Read the model definition and answer for the solid it produces. Units are mm, in the model's axes. A direction names the side the tool comes from. Give positions to 0.01 mm unless a question says otherwise; leave off trailing zeros. Write each loop counter-clockwise with the first axis right and the second up, starting at its lowest first coordinate (ties: lowest second). Pieces come first, ordered by that corner, then holes. Notation, with made-up numbers: M -31,35 L -8,35 A16 cw -8,61 Z; hole C -20,-15 d4. An arc over 180 degrees is marked long. Write each question's results on one line, items separated by ' | '. Start each with the question number.
```python
from build123d import *

# Parameters (mm, degrees)
SKETCH1_W                                 = 50.8
SKETCH1_H                                 = 63.5
BOSS_EXTRUDE1_DEPTH                       = 12.065
SKETCH6_W                                 = 50.8
SKETCH6_H                                 = 12.065
BOSS_EXTRUDE2_DEPTH                       = 6.35
F_13_64_0_20313_DIAMETER_HOLE1_AT_2_COUNT = 2
F_13_64_0_20313_DIAMETER_HOLE1_AT_2_PITCH = 31.75
SKETCH12_W                                = 25.4
SKETCH12_H                                = 50.8
CUT_EXTRUDE7_DEPTH                        = 48.353291596
FILLET1_R                                 = 6.35
SKETCH13_R                                = 19.05
CUT_EXTRUDE8_DEPTH                        = 48.353291596
FILLET2_R                                 = 6.35


with BuildPart() as part:
    # Sketch1 → Boss-Extrude1 (new body)
    with BuildSketch(Plane.XY):
        Rectangle(SKETCH1_W, SKETCH1_H)
    extrude(amount=BOSS_EXTRUDE1_DEPTH)

    # Sketch6 → Boss-Extrude2 (add)
    with BuildSketch(Plane.XZ.offset(31.75)):
        with Locations((0, 6.0325)):
            Rectangle(SKETCH6_W, SKETCH6_H)
    boss_extrude2 = extrude(amount=BOSS_EXTRUDE2_DEPTH)

    # Sketch8 → 13_64 _0.20313_ Diameter Hole1 (revolve, cut)
    with BuildSketch(Plane(origin=(-15.875, -38.1, 6.0325), x_dir=(0, 0, -1), z_dir=(1, 0, 0))):
        Polygon((0, 0), (0, 16.790070783), (2.579751, 15.24), (2.579751, 0), align=None)
    f_13_64_0_20313_diameter_hole1 = revolve(axis=Axis((-15.875, -44.45, 6.0325), (0, 1, 0)), mode=Mode.SUBTRACT)

    # 13_64 _0.20313_ Diameter Hole1 at 2: 13_64 _0.20313_ Diameter Hole1 ×2
    with Locations(*[(i * F_13_64_0_20313_DIAMETER_HOLE1_AT_2_PITCH, 0, 0) for i in range(1, F_13_64_0_20313_DIAMETER_HOLE1_AT_2_COUNT)]):
        add(f_13_64_0_20313_diameter_hole1, mode=Mode.SUBTRACT)

    # Mirror2: Boss-Extrude2, 13_64 _0.20313_ Diameter Hole1 across plane
    add(boss_extrude2.mirror(Plane.ZX))
    add(f_13_64_0_20313_diameter_hole1.mirror(Plane.ZX), mode=Mode.SUBTRACT)

    # Mirror2 copy 1 sketch → Mirror2 copy 1 (revolve, cut)
    with BuildSketch(Plane(origin=(15.875, 38.1, 6.0325), x_dir=(0, 0, -1), z_dir=(1, 0, 0))):
        Polygon((0, 0), (0, -16.790070783), (2.579751, -15.24), (2.579751, 0), align=None)
    revolve(axis=Axis((15.875, 44.45, 6.0325), (0, 1, 0)), mode=Mode.SUBTRACT)

    # Sketch12 → Cut-Extrude7 (cut, through all)
    with BuildSketch(Plane.XY.offset(12.065)):
        Rectangle(SKETCH12_W, SKETCH12_H)
    extrude(amount=-CUT_EXTRUDE7_DEPTH, mode=Mode.SUBTRACT)

    # Fillet1
    fillet1_edges = [part.edges().sort_by_distance(p)[0] for p in [
        (-12.7, -25.4, 6.0325),
        (-12.7, 25.4, 6.0325),
        (12.7, 25.4, 6.0325),
        (12.7, -25.4, 6.0325),
    ]]
    fillet(fillet1_edges, radius=FILLET1_R)

    # Sketch13 → Cut-Extrude8 (cut, through all)
    with BuildSketch(Plane(origin=(0, 0, 0), x_dir=(-1, 0, 0), z_dir=(0, 0, -1))):
        Circle(SKETCH13_R)
    extrude(amount=-CUT_EXTRUDE8_DEPTH, mode=Mode.SUBTRACT)

    # Fillet2
    fillet2_edges = [part.edges().sort_by_distance(p)[0] for p in [
        (12.7, 14.199031657, 6.0325),
        (12.7, -14.199031657, 6.0325),
        (-12.7, 14.199031657, 6.0325),
        (-12.7, -14.199031657, 6.0325),
    ]]
    fillet(fillet2_edges, radius=FILLET2_R)


solid = part.part
```
Item 1: For faces 5 (the flat face through (-17, -9, 0)), 6 (the flat face through (25.4, -1, 6)), 7 (the cylindrical face through (-18.05, -30.587, 4.646)), 8 (the flat face through (0, -25.4, 6)), 9 (the cylindrical face through (13.317, 30.587, 6.368)), determine the directions among +Z, -Z, +X, -X, +Y, -Y from which every point of the face is accessible in a straight line to the end or side of a thin tool.
Item 2: Section C-C, the plane z = 1.5 is taken. Determine the outline of the cut face in (x, y).
Item 3: Section D-D, the plane y = 27.5 is taken. Determine the outline of the cut face in (x, z) (1 decimal), then the cut area to 3 significant figures.
Item 4: Determine the mould class of faces 1 (the conical face through (-15.6, 21.58, 6.39)), 2 (the cylindrical face through (10.89, -23.49, 5.95)), 3 (the cylindrical face through (-18.05, 30.587, 4.646)), 4 (the flat face through (-17, -9, 12.065)) for opening direction Z: +Z half, -Z half, draft (parallel to the pull), parting line (faces both ways), or undercut.
Item 5: Section B-B, the plane y = 13.5 is taken. Determine the outline of the cut face in (x, z) (3 decimals), then the cut area to 3 significant figures.
Item 6: Straight lines are drawn through the part: line 1 (X direction, y = 18, z = 2.5); line 2 (X direction, y = -9, z = 5.25); line 3 (X direction, y = 24.5, z = 4). For each, find the intervals that lie inside material, in ascending order.
Item 7: Section A-A, the plane x = 9 is taken. Determine the outline of the cut face in (y, z) (3 decimals), then the cut area to 3 significant figures.
Item 8: Given P1, Ø3, axis at x = -15.88, z = 6.03, coming from the -Y side; P2, Ø4, axis at x = 15.88, z = 6.03, coming from the -Y side (3 decimals); P3, Ø4, axis at x = 15.88, z = 6.03, coming from the +Y side (3 decimals), each flat-ended and moving along its own axis, determine where each tip first touches the part or whether it passes through.
Worked out:
1) face 5: -Z, +X, -X, +Y, -Y | face 6: +Z, -Z, +X, +Y, -Y | face 7: -Y | face 8: +Z, -Z | face 9: +Y
2) outline: M -25.4,-38.1 L 25.4,-38.1 L 25.4,38.1 L -25.4,38.1 Z; hole M -14.29,-12.6 A6.35 cw -12.7,-16.8 L -12.7,-19.05 A6.35 ccw -6.35,-25.4 L 6.35,-25.4 A6.35 ccw 12.7,-19.05 L 12.7,-16.8 A6.35 cw 14.29,-12.6 A19.05 ccw 14.29,12.6 A6.35 cw 12.7,16.8 L 12.7,19.05 A6.35 ccw 6.35,25.4 L -6.35,25.4 A6.35 ccw -12.7,19.05 L -12.7,16.8 A6.35 cw -14.29,12.6 A19.05 ccw Z
3) outline: M -25.4,0 L 25.4,0 L 25.4,12.1 L -25.4,12.1 Z; hole C -15.9,6 d5.2; hole C 15.9,6 d5.2 | area: 571 mm²
4) face 1: undercut | face 2: draft | face 3: undercut | face 4: +Z half
5) outline: M -25.4,0 L -13.625,0 L -13.625,12.065 L -25.4,12.065 Z; M 13.625,0 L 25.4,0 L 25.4,12.065 L 13.625,12.065 Z | area: 284 mm²
6) line 1: x = -25.4 to -12.7, 12.7 to 25.4 | line 2: x = -25.4 to -16.79, 16.79 to 25.4 | line 3: x = -25.4 to -17.46, -14.29 to -9.61, 9.61 to 14.29, 17.46 to 25.4
7) outline: M -38.1,0 L -24.821,0 L -24.821,12.065 L -38.1,12.065 Z; M 24.821,0 L 38.1,0 L 38.1,12.065 L 24.821,12.065 Z | area: 320 mm²
8) P1: stops at y = -22.21 | P2: stops at y = -22.515 | P3: stops at y = 22.515
